from build123d import *

# Parameters (mm, degrees)
SKETCH_1_W          = 8
SKETCH_1_H          = 35.5
EXTRUDE_1_DEPTH     = 10
CUT_EXTRUDE_1_REACH = 22.762
SKETCH_2_R          = 1.65
SKETCH_3_R          = 3
CUT_EXTRUDE_2_DEPTH = 7


with BuildPart() as part:
    # 草图1 → 凸台-拉伸1 (new body)
    with BuildSketch(Plane(origin=(0, 0, 0), x_dir=(1, 0, 0), z_dir=(0, 1, 0))):
        Rectangle(SKETCH_1_W, SKETCH_1_H)
    extrude(amount=EXTRUDE_1_DEPTH)

    # 草图2 → 切除-拉伸1 (cut, up to next)
    with BuildSketch(Plane(origin=(0, 10, 0), x_dir=(1, 0, 0), z_dir=(0, 1, 0)), mode=Mode.PRIVATE) as cut_extrude_1_sk1:
        with Locations(Location((0, 12.5, 0), (0, 0, 270))):
            Circle(SKETCH_2_R)
    cut_extrude_1_tool1 = extrude(cut_extrude_1_sk1.sketch, amount=-CUT_EXTRUDE_1_REACH, mode=Mode.PRIVATE) & part.part
    # 草图2 → 切除-拉伸1 (cut, up to next)
    with BuildSketch(Plane(origin=(0, 10, 0), x_dir=(1, 0, 0), z_dir=(0, 1, 0)), mode=Mode.PRIVATE) as cut_extrude_1_sk2:
        with Locations(Location((0, -12.5, 0), (0, 0, 270))):
            Circle(SKETCH_2_R)
    cut_extrude_1_tool2 = extrude(cut_extrude_1_sk2.sketch, amount=-CUT_EXTRUDE_1_REACH, mode=Mode.PRIVATE) & part.part
    add(cut_extrude_1_tool1.solids().sort_by_distance((0, 10, -12.5))[0], mode=Mode.SUBTRACT)
    add(cut_extrude_1_tool2.solids().sort_by_distance((0, 10, 12.5))[0], mode=Mode.SUBTRACT)

    # 草图3 → 切除-拉伸2 (cut)
    with BuildSketch(Plane(origin=(0, 0, 0), x_dir=(1, 0, 0), z_dir=(0, 1, 0))):
        with Locations(Location((0, 12.5, 0), (0, 0, 270))):
            Circle(SKETCH_3_R)
        with Locations(Location((0, -12.5, 0), (0, 0, 270))):
            Circle(SKETCH_3_R)
    extrude(amount=CUT_EXTRUDE_2_DEPTH, mode=Mode.SUBTRACT)


solid = part.part
Can you work these out from the model? Positions are in its coordinate system, mm. A direction names the side the tool comes from. Give positions to 0.01 mm unless a question says otherwise; leave off trailing zeros. Order: outer loops, then holes, each group sorted by start corner. A loop starts at its lowest first (then second) coordinate and runs counter-clockwise, first axis right, second up. Notation, with made-up numbers: M -34.75,-40 L -6.75,-40 A14 ccw -6.75,-16 Z; hole C -30,-28 d7. An arc over 180 degrees is marked long. Use a Markdown table: item, result. Add a question column.
Item 1: Suppose I cut it at A-A (x = 0). List the corners of the cut face in (y, z) for me.
Item 2: If I drill on L1, parallel to X at y = 7.8, z = -12.5; L2, parallel to Z at x = 2.5, y = 6.25; L3, parallel to Z at x = 0.25, y = 2, over which ranges is the centre line in solid material (lowest first)? Write a range as [from, to].
Item 3: Will this pin go through, and if not, where does the flat tip stop? pin 1 (4.5 mm diameter, centred on x = 0, z = -12.5, fed in from -Y).
Item 4: Suppose I cut it at C-C (y = 4.5). List the corners of the cut face in (x, z) for me, then the cut area to 3 significant figures.
Item 5: We'd pull the mould along Z, two halves only. Please class faces 3 (the flat face through (0, 5, -17.75)), 4 (the cylindrical face through (0.1, 3.5, 9.5)), 5 (the flat face through (0, 10, 0)): +Z half, -Z half, draft (parallel to the pull), parting line (faces both ways), or undercut.
Item 6: For faces 1 (the cylindrical face through (0.1, 3.5, -15.5)), 2 (the flat face through (0, 5, 17.75)), which set-ups out of +Z, -Z, +X, -X, +Y, -Y let a thin tool reach every point of the face, with its end or its side?
Item 7: Suppose I cut it at B-B (z = -12.5). List the corners of the cut face in (x, y) for me.
Item 8: Suppose I cut it at D-D (x = -2). List the corners of the cut face in (y, z) for me, then the cut area to 3 significant figures.
Answer sheet:
| question | item | result |
|---|---|---|
| 1 | outline | M 0,-17.75 L 10,-17.75 L 10,-14.15 L 7,-14.15 L 7,-15.5 L 0,-15.5 Z; M 0,-9.5 L 7,-9.5 L 7,-10.85 L 10,-10.85 L 10,10.85 L 7,10.85 L 7,9.5 L 0,9.5 Z; M 0,15.5 L 7,15.5 L 7,14.15 L 10,14.15 L 10,17.75 L 0,17.75 Z |
| 2 | L1 | x = [-4, -1.65], [1.65, 4] |
| 2 | L2 | z = [-17.75, -14.16], [-10.84, 10.84], [14.16, 17.75] |
| 2 | L3 | z = [-17.75, -15.49], [-9.51, 9.51], [15.49, 17.75] |
| 3 | pin 1 | stops at y = 7 |
| 4 | outline | M -4,-17.75 L 4,-17.75 L 4,17.75 L -4,17.75 Z; hole C 0,-12.5 d6; hole C 0,12.5 d6 |
| 4 | area | 227 mm² |
| 5 | face 3 | -Z half |
| 5 | face 4 | undercut |
| 5 | face 5 | draft |
| 6 | face 1 | -Y |
| 6 | face 2 | +Z, +X, -X, +Y, -Y |
| 7 | outline | M -4,0 L -3,0 L -3,7 L -1.65,7 L -1.65,10 L -4,10 Z; M 1.65,7 L 3,7 L 3,0 L 4,0 L 4,10 L 1.65,10 Z |
| 8 | outline | M 0,-17.75 L 10,-17.75 L 10,17.75 L 0,17.75 L 0,14.74 L 7,14.74 L 7,10.26 L 0,10.26 L 0,-10.26 L 7,-10.26 L 7,-14.74 L 0,-14.74 Z |
| 8 | area | 292 mm² |
